For this review, take the finished solid that the model builds, in its own axes (mm). A direction names the side the tool comes from. Round coordinates to 2 decimals unless told otherwise and drop trailing zeros. Loops run counter-clockwise (first coordinate to the right, second up) from the corner with the lowest first, then second, coordinate; pieces in that order, holes last.
```python
from build123d import *

# Parameters (mm, degrees)
SKETCH_W          = 32
SKETCH_H          = 15
PAD_DEPTH         = 24
SKETCH001_W       = 7.5
SKETCH001_H       = 15
SKETCH002_R       = 1.525
HOLE_DEPTH        = 25
POCKET_DEPTH      = 7.501
POCKET_DEPTH_BACK = -7.501
POCKET001_DEPTH   = 19
FILLET_R          = 1.5


with BuildPart() as part:
    # Sketch → Pad (new body)
    with BuildSketch(Plane.XY):
        Rectangle(SKETCH_W, SKETCH_H)
    extrude(amount=PAD_DEPTH)

    # Sketch001 → Groove (revolve, cut)
    with BuildSketch(Plane.XY.offset(12)):
        with Locations((-3.75, 0)):
            Rectangle(SKETCH001_W, SKETCH001_H)
    revolve(axis=Axis((0, 0, 12), (0, 1, 0)), mode=Mode.SUBTRACT)

    # Sketch002 → Hole (cut)
    with BuildSketch(Plane.XY.offset(24)):
        with Locations((12, 0)):
            Circle(SKETCH002_R)
        with Locations((-12, 0)):
            Circle(SKETCH002_R)
    extrude(amount=-HOLE_DEPTH, mode=Mode.SUBTRACT)

    # Sketch004 → Pocket (cut, two sides)
    with BuildSketch(Plane.XZ) as pocket_sk:
        with BuildLine():
            Line((-25, 7), (-14.866069, 7))
            ThreePointArc((-14.866069, 7), (-12.607751, 8.025158), (-11.892855, 10.4))
            ThreePointArc((11.892855, 10.4), (0, 24), (-11.892855, 10.4))
            ThreePointArc((11.892855, 10.4), (12.607751, 8.025158), (14.866069, 7))
            Line((14.866069, 7), (25, 7))
            Line((25, 7), (25, 37.147858))
            Line((25, 37.147858), (-25, 37.147858))
            Line((-25, 7), (-25, 37.147858))
        make_face()
    extrude(amount=-POCKET_DEPTH, mode=Mode.SUBTRACT)
    extrude(pocket_sk.sketch, amount=-POCKET_DEPTH_BACK, mode=Mode.SUBTRACT)

    # Sketch003 → Pocket001 (cut)
    with BuildSketch(Plane.XY.offset(24)):
        Polygon((14.65, 1.529978), (12, 3.059956), (9.35, 1.529978), (9.35, -1.529978), (12, -3.059956), (14.65, -1.529978), align=None)
        Polygon((-9.35, 1.529978), (-12, 3.059956), (-14.65, 1.529978), (-14.65, -1.529978), (-12, -3.059956), (-9.35, -1.529978), align=None)
    extrude(amount=-POCKET001_DEPTH, mode=Mode.SUBTRACT)

    # Fillet
    fillet_edges = [part.edges().sort_by_distance(p)[0] for p in [
        (16, 0, 7),
        (-16, 0, 7),
    ]]
    fillet(fillet_edges, radius=FILLET_R)


solid = part.part
```
(1) The part is to be moulded in two halves that separate along Z. For faces 1 (the flat face through (-13.049, -2.454, 6.171)), 2 (the flat face through (10.8, -1.3, 5)), 3 (the cylindrical face through (-12.551, -5.226, 8.092)), say which applies: pulls with the +Z half, pulls with the -Z half, needs draft (parallel to the pull), parting line crosses it, or undercut.
(2) Add section C-C (z = 8). Give the boundary of the cut face in (x, y).
(3) For L1, parallel to Y at x = 12, z = 1.9 (3 decimals); L2, parallel to X at y = 0.5, z = 1.25; L3, parallel to X at y = -0.25, z = 3.5, list the stretches that pass through material, from the lowest coordinate up.
(4) Add section B-B (y = 0). Give the number of separate pieces and of enclosed holes in the cut face, plus the area to 3 significant figures.
(5) Insertion check: pin 1 Ø1 at (x, z) = (-2.5, 7.5) entering from -Y; pin 2 Ø6 at (x, y) = (5, -3.5) entering from +Z; pin 3 Ø2.5 at (y, z) = (0, 13.5) entering from -X; pin 4 Ø1.5 at (x, y) = (-10.5, -1.5) entering from +Z. Each pin has a flat end and moves straight along its axis. Give the tip position at first contact, or say it passes through.
(6) For faces 4 (the flat face through (10.694, 2.306, 10.749)), 5 (the cylindrical face through (-12.551, 5.143, 8.092)), list the 3-axis set-ups (+Z, -Z, +X, -X, +Y, -Y) from which the entire face can be reached by the end or side of a thin tool; tool diameter is ignored.
(7) Add section D-D (x = 5.5). Give the boundary of the cut face in (y, z), plus the area to 3 significant figures.
(8) Add section A-A (x = 0). Give the boundary of the cut face in (y, z), plus the area to 3 significant figures.
Outcome:
1. face 1: needs draft
1. face 2: pulls with the +Z half
1. face 3: undercut
2. outline: (-12.63, -7.5) - (-6.34, -7.5) - (-6.34, 7.5) - (-12.63, 7.5) - (-12.63, 2.7) - (-12, 3.06) - (-9.35, 1.53) - (-9.35, -1.53) - (-12, -3.06) - (-12.63, -2.7) - close; (6.34, -7.5) - (12.63, -7.5) - (12.63, -2.7) - (12, -3.06) - (9.35, -1.53) - (9.35, 1.53) - (12, 3.06) - (12.63, 2.7) - (12.63, 7.5) - (6.34, 7.5) - close
3. L1: y = -7.5 to -1.525, 1.525 to 7.5
3. L2: x = -16 to -13.44, -10.56 to 10.56, 13.44 to 16
3. L3: x = -16 to -13.5, -10.5 to 10.5, 13.5 to 16
4. separate pieces: 3
4. enclosed holes: 1
4. area: 287 mm2
5. pin 1: passes through
5. pin 2: stops at z = 23.83
5. pin 3: stops at x = -9.35
5. pin 4: stops at z = 18.91
6. face 4: +Z
6. face 5: -X, +Y, -Y
7. outline: (-7.5, 0) - (7.5, 0) - (7.5, 6.9) - (-7.5, 6.9) - close; (-7.5, 17.1) - (7.5, 17.1) - (7.5, 22.67) - (-7.5, 22.67) - close
7. area: 187 mm2
8. outline: (-7.5, 0) - (7.5, 0) - (7.5, 4.5) - (-7.5, 4.5) - close; (-7.5, 19.5) - (7.5, 19.5) - (7.5, 24) - (-7.5, 24) - close
8. area: 135 mm2
